```python
from build123d import *

# Parameters (mm, degrees)
BOSS_EXTRUDE1_DEPTH = 7.5
FILLET1_R           = 10
SKETCH2_R           = 4.975
CUT_EXTRUDE1_DEPTH  = 7.5
CHAMFER1_SIZE       = 1.5


with BuildPart() as part:
    # Sketch1 → Boss-Extrude1 (new body)
    with BuildSketch(Plane(origin=(0, 0, 0), x_dir=(1, 0, 0), z_dir=(0, 1, 0))):
        Polygon((60, 0), (20, 0), (20, -20), (0, -20), (0, -60), (20, -60), (20, -80), (60, -80), (60, -60), (80, -60), (80, -20), (60, -20), align=None)
    extrude(amount=BOSS_EXTRUDE1_DEPTH)

    # Fillet1
    # the kernel refuses this fillet: 10 mm, written as the material it takes off along each edge
    with BuildSketch(Plane(origin=(20, 7.5, -24.206145914), x_dir=(0, -1, 0), z_dir=(0, 0, 1)), Plane(origin=(60, 7.5, 20), x_dir=(0, -1, 0), z_dir=(0, 0, -1)), Plane(origin=(104.206145914, 7.5, 20), x_dir=(0, -1, 0), z_dir=(-1, 0, 0)), Plane(origin=(60, 7.5, 60), x_dir=(0, -1, 0), z_dir=(1, 0, 0)), Plane(origin=(60, 7.5, 104.206145914), x_dir=(0, -1, 0), z_dir=(0, 0, -1)), Plane(origin=(20, 7.5, 60), x_dir=(0, -1, 0), z_dir=(0, 0, 1)), Plane(origin=(-24.206145914, 7.5, 60), x_dir=(0, -1, 0), z_dir=(1, 0, 0)), Plane(origin=(20, 7.5, 20), x_dir=(0, -1, 0), z_dir=(-1, 0, 0))) as fillet1_piece_1:
        with BuildLine():
            CenterArc((10, 9.682458366), FILLET1_R, 180, 75.522487814)
            Line((0, 9.682458366), (-0.2, 9.682458366))
            Line((-0.2, 9.682458366), (-0.2, 0))
            Line((-0.2, 0), (0, -0.2))
            ThreePointArc((0, -0.2), (3.75, -0.2), (7.45, -0.193649167))
            Line((7.45, -0.193649167), (7.5, 0))
        make_face()
    extrude(amount=44.206145914, mode=Mode.SUBTRACT)
    with BuildSketch(Plane(origin=(84.206145914, 7.5, 0), x_dir=(0, -1, 0), z_dir=(-1, 0, 0)), Plane(origin=(80, 7.5, 84.206145914), x_dir=(0, -1, 0), z_dir=(0, 0, -1)), Plane(origin=(-4.206145914, 7.5, 80), x_dir=(0, -1, 0), z_dir=(1, 0, 0)), Plane(origin=(0, 7.5, -4.206145914), x_dir=(0, -1, 0), z_dir=(0, 0, 1))) as fillet1_piece_2:
        with BuildLine():
            CenterArc((10, 9.682458366), FILLET1_R, 180, 75.522487814)
            Line((0, 9.682458366), (-0.2, 9.682458366))
            Line((-0.2, 9.682458366), (-0.2, 0))
            Line((-0.2, 0), (0, -0.2))
            ThreePointArc((0, -0.2), (3.75, -0.2), (7.45, -0.193649167))
            Line((7.45, -0.193649167), (7.5, 0))
        make_face()
    extrude(amount=88.412291828, mode=Mode.SUBTRACT)
    with BuildSketch(Plane(origin=(20, 7.5, -24.206145914), x_dir=(0, -1, 0), z_dir=(0, 0, 1))) as fillet1_piece_3a_section:
        with BuildLine():
            CenterArc((10, 9.682458366), FILLET1_R, 180, 75.522487814)
            Line((0, 9.682458366), (-0.2, 9.682458366))
            Line((-0.2, 9.682458366), (-0.2, 0))
            Line((-0.2, 0), (0, -0.2))
            ThreePointArc((0, -0.2), (3.75, -0.2), (7.45, -0.193649167))
            Line((7.45, -0.193649167), (7.5, 0))
        make_face()
    fillet1_piece_3a = extrude(amount=68.412291828, mode=Mode.PRIVATE)
    fillet1_piece_3a = split(fillet1_piece_3a, bisect_by=Plane(origin=(22.281441008, 5.604082443, 20), z_dir=(0, 0, 1)), keep=Keep.TOP, mode=Mode.PRIVATE)
    with BuildSketch(Plane(origin=(44.206145914, 7.5, 20), x_dir=(0, -1, 0), z_dir=(-1, 0, 0))) as fillet1_piece_3b_section:
        with BuildLine():
            CenterArc((10, 9.682458366), FILLET1_R, 180, 75.522487814)
            Line((0, 9.682458366), (-0.2, 9.682458366))
            Line((-0.2, 9.682458366), (-0.2, 0))
            Line((-0.2, 0), (0, -0.2))
            ThreePointArc((0, -0.2), (3.75, -0.2), (7.45, -0.193649167))
            Line((7.45, -0.193649167), (7.5, 0))
        make_face()
    fillet1_piece_3b = extrude(amount=68.412291828, mode=Mode.PRIVATE)
    fillet1_piece_3b = split(fillet1_piece_3b, bisect_by=Plane(origin=(20, 5.604082443, 22.281441008), z_dir=(1, 0, 0)), keep=Keep.TOP, mode=Mode.PRIVATE)
    fillet1_piece_3 = fillet1_piece_3a & fillet1_piece_3b
    add(fillet1_piece_3, mode=Mode.SUBTRACT)
    with BuildSketch(Plane(origin=(104.206145914, 7.5, 20), x_dir=(0, -1, 0), z_dir=(-1, 0, 0))) as fillet1_piece_4a_section:
        with BuildLine():
            CenterArc((10, 9.682458366), FILLET1_R, 180, 75.522487814)
            Line((0, 9.682458366), (-0.2, 9.682458366))
            Line((-0.2, 9.682458366), (-0.2, 0))
            Line((-0.2, 0), (0, -0.2))
            ThreePointArc((0, -0.2), (3.75, -0.2), (7.45, -0.193649167))
            Line((7.45, -0.193649167), (7.5, 0))
        make_face()
    fillet1_piece_4a = extrude(amount=68.412291828, mode=Mode.PRIVATE)
    fillet1_piece_4a = split(fillet1_piece_4a, bisect_by=Plane(origin=(60, 5.604082443, 22.281441008), z_dir=(-1, 0, 0)), keep=Keep.TOP, mode=Mode.PRIVATE)
    with BuildSketch(Plane(origin=(60, 7.5, 44.206145914), x_dir=(0, -1, 0), z_dir=(0, 0, -1))) as fillet1_piece_4b_section:
        with BuildLine():
            CenterArc((10, 9.682458366), FILLET1_R, 180, 75.522487814)
            Line((0, 9.682458366), (-0.2, 9.682458366))
            Line((-0.2, 9.682458366), (-0.2, 0))
            Line((-0.2, 0), (0, -0.2))
            ThreePointArc((0, -0.2), (3.75, -0.2), (7.45, -0.193649167))
            Line((7.45, -0.193649167), (7.5, 0))
        make_face()
    fillet1_piece_4b = extrude(amount=68.412291828, mode=Mode.PRIVATE)
    fillet1_piece_4b = split(fillet1_piece_4b, bisect_by=Plane(origin=(57.718558992, 5.604082443, 20), z_dir=(0, 0, 1)), keep=Keep.TOP, mode=Mode.PRIVATE)
    fillet1_piece_4 = fillet1_piece_4a & fillet1_piece_4b
    add(fillet1_piece_4, mode=Mode.SUBTRACT)
    with BuildSketch(Plane(origin=(60, 7.5, 104.206145914), x_dir=(0, -1, 0), z_dir=(0, 0, -1))) as fillet1_piece_5a_section:
        with BuildLine():
            CenterArc((10, 9.682458366), FILLET1_R, 180, 75.522487814)
            Line((0, 9.682458366), (-0.2, 9.682458366))
            Line((-0.2, 9.682458366), (-0.2, 0))
            Line((-0.2, 0), (0, -0.2))
            ThreePointArc((0, -0.2), (3.75, -0.2), (7.45, -0.193649167))
            Line((7.45, -0.193649167), (7.5, 0))
        make_face()
    fillet1_piece_5a = extrude(amount=68.412291828, mode=Mode.PRIVATE)
    fillet1_piece_5a = split(fillet1_piece_5a, bisect_by=Plane(origin=(57.718558992, 5.604082443, 60), z_dir=(0, 0, -1)), keep=Keep.TOP, mode=Mode.PRIVATE)
    with BuildSketch(Plane(origin=(35.793854086, 7.5, 60), x_dir=(0, -1, 0), z_dir=(1, 0, 0))) as fillet1_piece_5b_section:
        with BuildLine():
            CenterArc((10, 9.682458366), FILLET1_R, 180, 75.522487814)
            Line((0, 9.682458366), (-0.2, 9.682458366))
            Line((-0.2, 9.682458366), (-0.2, 0))
            Line((-0.2, 0), (0, -0.2))
            ThreePointArc((0, -0.2), (3.75, -0.2), (7.45, -0.193649167))
            Line((7.45, -0.193649167), (7.5, 0))
        make_face()
    fillet1_piece_5b = extrude(amount=68.412291828, mode=Mode.PRIVATE)
    fillet1_piece_5b = split(fillet1_piece_5b, bisect_by=Plane(origin=(60, 5.604082443, 57.718558992), z_dir=(-1, 0, 0)), keep=Keep.TOP, mode=Mode.PRIVATE)
    fillet1_piece_5 = fillet1_piece_5a & fillet1_piece_5b
    add(fillet1_piece_5, mode=Mode.SUBTRACT)
    with BuildSketch(Plane(origin=(-24.206145914, 7.5, 60), x_dir=(0, -1, 0), z_dir=(1, 0, 0))) as fillet1_piece_6a_section:
        with BuildLine():
            CenterArc((10, 9.682458366), FILLET1_R, 180, 75.522487814)
            Line((0, 9.682458366), (-0.2, 9.682458366))
            Line((-0.2, 9.682458366), (-0.2, 0))
            Line((-0.2, 0), (0, -0.2))
            ThreePointArc((0, -0.2), (3.75, -0.2), (7.45, -0.193649167))
            Line((7.45, -0.193649167), (7.5, 0))
        make_face()
    fillet1_piece_6a = extrude(amount=68.412291828, mode=Mode.PRIVATE)
    fillet1_piece_6a = split(fillet1_piece_6a, bisect_by=Plane(origin=(20, 5.604082443, 57.718558992), z_dir=(1, 0, 0)), keep=Keep.TOP, mode=Mode.PRIVATE)
    with BuildSketch(Plane(origin=(20, 7.5, 35.793854086), x_dir=(0, -1, 0), z_dir=(0, 0, 1))) as fillet1_piece_6b_section:
        with BuildLine():
            CenterArc((10, 9.682458366), FILLET1_R, 180, 75.522487814)
            Line((0, 9.682458366), (-0.2, 9.682458366))
            Line((-0.2, 9.682458366), (-0.2, 0))
            Line((-0.2, 0), (0, -0.2))
            ThreePointArc((0, -0.2), (3.75, -0.2), (7.45, -0.193649167))
            Line((7.45, -0.193649167), (7.5, 0))
        make_face()
    fillet1_piece_6b = extrude(amount=68.412291828, mode=Mode.PRIVATE)
    fillet1_piece_6b = split(fillet1_piece_6b, bisect_by=Plane(origin=(22.281441008, 5.604082443, 60), z_dir=(0, 0, -1)), keep=Keep.TOP, mode=Mode.PRIVATE)
    fillet1_piece_6 = fillet1_piece_6a & fillet1_piece_6b
    add(fillet1_piece_6, mode=Mode.SUBTRACT)

    # Sketch2 → Cut-Extrude1 (cut)
    with BuildSketch(Plane(origin=(0, 0, 0), x_dir=(1, 0, 0), z_dir=(0, 1, 0))):
        with Locations(Location((40, -40, 0), (0, 0, 270))):
            Circle(SKETCH2_R)
    extrude(amount=CUT_EXTRUDE1_DEPTH, mode=Mode.SUBTRACT)

    # Chamfer1
    chamfer1_edges = [part.edges().sort_by_distance(p)[0] for p in [
        (40, 0, 35.025),
    ]]
    chamfer(chamfer1_edges, length=CHAMFER1_SIZE)


solid = part.part
```
Can you work these out from the model? Positions are in its coordinate system, mm. A direction names the side the tool comes from. Give positions to 0.01 mm unless a question says otherwise; leave off trailing zeros. Write each loop counter-clockwise with the first axis right and the second up, starting at its lowest first coordinate (ties: lowest second). Pieces come first, ordered by that corner, then holes. Notation, with made-up numbers: (-2, 67) -> (52, 67) arc R19 cw to (52, 73) -> close; hole circle Ø2 at (45.5, -27). An arc over 180 degrees is marked (long way). Write item = value, one per line.
(1) I need wall thicknesses on probe 1 along Z at (x, y) = (43, 5.25); probe 2 along X at (y, z) = (6.1, 40) (3 decimals); probe 3 along X at (y, z) = (5.5, 40) (3 decimals). Which ranges of each line are inside material? Lowest first, please. Write a range as from..to.
Worked out:
probe_1 = 3.36..36.03, 43.97..76.64
probe_2 = 4.58..35.025, 44.975..75.42
probe_3 = 3.682..35.025, 44.975..76.318
(2) Suppose I cut it at A-A on z = 40. Write out the boundary of the cut face in (x, y) (3 decimals).
Worked out:
outline = (0, 0) -> (33.525, 0) -> (35.025, 1.5) -> (35.025, 7.5) -> (9.682, 7.5) arc R10 ccw to start; (44.975, 1.5) -> (46.475, 0) -> (80, 0) arc R10 ccw to (70.318, 7.5) -> (44.975, 7.5) -> close
(3) I'm going to push flat-ended pins straight in: P1, Ø1, axis at y = 3.5, z = 22, coming from the -X side; P2, Ø2, axis at y = 3, z = 12, coming from the +X side; P3, Ø8, axis at x = 40, z = 40, coming from the -Y side; P4, Ø1.5, axis at x = 60, y = 2.5, coming from the +Z side. Where does each tip first touch, or does it pass through?
Worked out:
P1 = 1.33
P2 = 59.25
P3 = through
P4 = 59.37
(4) Suppose I cut it at D-D on x = 57. Write out the boundary of the cut face in (y, z).
Worked out:
outline = (0, 0) arc R10 ccw to (4.94, 3) -> (4.94, 23) arc R10 ccw to (7.5, 29.68) -> (7.5, 50.32) arc R10 ccw to (4.94, 57) -> (4.94, 77) arc R10 ccw to (0, 80) -> close
(5) For faces 5 (the face through (23.63, 5.46, 64.95)), 6 (the face through (15.05, 5.46, 23.63)), 7 (the face through (64.95, 5.46, 56.37)), 8 (the face through (65.37, 5.46, 23.63)), which set-ups out of +Z, -Z, +X, -X, +Y, -Y let a thin tool reach every point of the face, with its end or its side?
Worked out:
face_5 = +Z, -X, +Y
face_6 = -Z, -X, +Y
face_7 = +Z, +X, +Y
face_8 = -Z, +X, +Y
(6) Suppose I cut it at B-B on x = 40. Write out the boundary of the cut face in (y, z) (3 decimals).
Worked out:
outline = (0, 0) arc R10 ccw to (7.5, 9.682) -> (7.5, 35.025) -> (1.5, 35.025) -> (0, 33.525) -> close; (0, 46.475) -> (1.5, 44.975) -> (7.5, 44.975) -> (7.5, 70.318) arc R10 ccw to (0, 80) -> close
(7) Suppose I cut it at C-C on y = 5.5. Write out the boundary of the cut face in (x, z) (3 decimals).
Worked out:
outline = (3.682, 23.682) -> (23.682, 23.682) -> (23.682, 3.682) -> (56.318, 3.682) -> (56.318, 23.682) -> (76.318, 23.682) -> (76.318, 56.318) -> (56.318, 56.318) -> (56.318, 76.318) -> (23.682, 76.318) -> (23.682, 56.318) -> (3.682, 56.318) -> close; hole circle Ø9.95 at (40, 40)
(8) Thinking about a two-plate mould opening in X: for faces 1 (the face through (40, 7.5, 46)), 2 (the face through (2.53, 4.49, 39.72)), 3 (the face through (36.973, 4.458, 36.052)), 4 (the face through (56.37, 5.46, 65.37)), which applies, released by +X, released by -X, zero draft, split by the parting line, or undercut?
Worked out:
face_1 = zero draft
face_2 = released by -X
face_3 = undercut
face_4 = released by +X
